Geometry: final body of the model. Coordinates: model frame, mm. Face numbers are marked on the shaded views. A direction names the side the tool comes from. Give positions to 0.01 mm unless a question says otherwise; leave off trailing zeros. Order: outer loops, then holes, each group sorted by start corner. A loop starts at its lowest first (then second) coordinate and runs counter-clockwise, first axis right, second up. Notation, with made-up numbers: M -37,7.5 L -29,7.5 A25 cw -29,23.5 Z; hole C -31,69.5 d1. An arc over 180 degrees is marked long. Use CSV: the item, a comma, the result in double quotes.
```python
from build123d import *

# Parameters (mm, degrees)
PAD_DEPTH       = 4.5
SKETCH001_R     = 3.6
POCKET_DEPTH    = 4.501
POCKET001_DEPTH = 1.5
SKETCH003_R     = 0.6
POCKET002_DEPTH = 3.001
CHAMFER_SIZE    = 0.6


with BuildPart() as part:
    # Sketch → Pad (new body)
    with BuildSketch(Plane.XY):
        with BuildLine():
            ThreePointArc((0, -4.5), (4.5, 0), (0, 4.5))
            Line((0, 4.5), (-26, 4.5))
            ThreePointArc((-26, 4.5), (-29.181981, 3.181981), (-30.5, 0))
            ThreePointArc((-30.5, 0), (-23.829371, -8.693332), (-13.705771, -4.5))
            Line((0, -4.5), (-13.705771, -4.5))
        make_face()
    extrude(amount=PAD_DEPTH)

    # Sketch001 (on Face7 of Pad) → Pocket (cut, through all)
    with BuildSketch(Plane.XY.offset(4.5)):
        Circle(SKETCH001_R)
    extrude(amount=-POCKET_DEPTH, mode=Mode.SUBTRACT)

    # Sketch002 (on Face5 of Pocket) → Pocket001 (cut)
    with BuildSketch(Plane.XY.offset(4.5)):
        with BuildLine():
            ThreePointArc((-14.63696, 1.995305), (-16.5, 0), (-14.63696, -1.995305))
            Line((-14.63696, -1.995305), (0, -3))
            Line((0, 3), (0, -3))
            Line((-14.63696, 1.995305), (0, 3))
        make_face()
    extrude(amount=-POCKET001_DEPTH, mode=Mode.SUBTRACT)

    # Sketch003 (on Face12 of Pocket001) → Pocket002 (cut, through all)
    with BuildSketch(Plane.XY.offset(3)):
        with Locations((-14.5, 0)):
            Circle(SKETCH003_R)
        with Locations((-12.5, 0)):
            Circle(SKETCH003_R)
        with Locations((-10.5, 0)):
            Circle(SKETCH003_R)
        with Locations((-8.5, 0)):
            Circle(SKETCH003_R)
        with Locations((-6.5, 0)):
            Circle(SKETCH003_R)
        with Locations((-4.5, 0)):
            Circle(SKETCH003_R)
    extrude(amount=-POCKET002_DEPTH, mode=Mode.SUBTRACT)

    # Chamfer
    chamfer_edges = [part.edges().sort_by_distance(p)[0] for p in [
        (-23.829371, -8.693332, 4.5),
        (-23.829371, -8.693332, 0),
    ]]
    chamfer(chamfer_edges, length=CHAMFER_SIZE)


solid = part.part
```
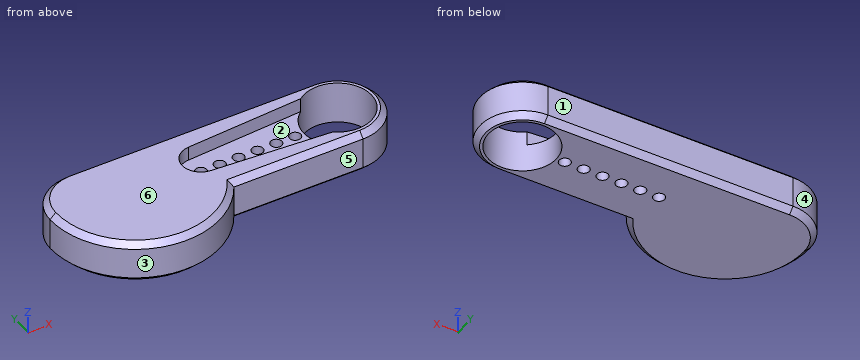
1. Pull-direction query (X, two-part tool) for the marked faces 1, 2, 3 and 4; classes: +X half, -X half, draft (parallel to the pull), parting line (faces both ways), or undercut.
Answer:
face 1,"draft"
face 2,"undercut"
face 3,"parting line"
face 4,"-X half"
2. Section D-D, the plane x = -6.5. Return the cut outline in (y, z), plus the area to 3 significant figures.
Answer:
outline,"M -4.5,0.6 L -3.9,0 L -0.6,0 L -0.6,3 L -2.55,3 L -2.55,4.5 L -3.9,4.5 L -4.5,3.9 Z; M 0.6,0 L 3.9,0 L 4.5,0.6 L 4.5,3.9 L 3.9,4.5 L 2.55,4.5 L 2.55,3 L 0.6,3 Z"
area,"28.5 mm2"
3. Section C-C, the plane x = -1. Return the cut outline in (y, z), plus the area to 3 significant figures.
Answer:
outline,"M -4.5,0.6 L -3.9,0 L -3.46,0 L -3.46,4.5 L -3.9,4.5 L -4.5,3.9 Z; M 3.46,0 L 3.9,0 L 4.5,0.6 L 4.5,3.9 L 3.9,4.5 L 3.46,4.5 Z"
area,"8.66 mm2"
4. Section B-B, the plane x = -10.5. Return the cut outline in (y, z), plus the area to 3 significant figures.
Answer:
outline,"M -4.5,0.6 L -3.9,0 L -0.6,0 L -0.6,3 L -2.28,3 L -2.28,4.5 L -3.9,4.5 L -4.5,3.9 Z; M 0.6,0 L 3.9,0 L 4.5,0.6 L 4.5,3.9 L 3.9,4.5 L 2.28,4.5 L 2.28,3 L 0.6,3 Z"
area,"29.3 mm2"
5. Pin query (flat end, axial travel): pin 1 Ø0.7 at (x, y) = (-4.5, 0) entering from +Z; pin 2 Ø1.4 at (x, y) = (-14.5, 0) entering from +Z; pin 3 Ø2 at (x, z) = (-6.5, 1) entering from -Y. Return the tip coordinate at first contact, or that it passes through.
Answer:
pin 1,"through"
pin 2,"z = 3"
pin 3,"y = -4.5"
6. Reachability of the marked faces 5 and 6 from +Z, -Z, +X, -X, +Y, -Y: full face, straight path, thin tool, end or side. Return the list, or none.
Answer:
face 5,"+Z, -Z, +X, -Y"
face 6,"+Z, +X, -X, +Y, -Y"
7. Section A-A, the plane z = 1.2. Return the cut outline in (x, y), plus the area to 3 significant figures.
Answer:
outline,"M -30.5,0 A9 ccw -13.71,-4.5 L 0,-4.5 A4.5 ccw 0,4.5 L -26,4.5 A4.5 ccw Z; hole C -14.5,0 d1.2; hole C -12.5,0 d1.2; hole C -10.5,0 d1.2; hole C -8.5,0 d1.2; hole C -6.5,0 d1.2; hole C -4.5,0 d1.2; hole C 0,0 d7.2"
area,"302 mm2"
8. Line query: line 1 (Y direction, x = -10.5, z = 1); line 2 (X direction, y = -1.5, z = 2.15); line 3 (X direction, y = 1.25, z = 3.35). Output: solid intervals per line, ascending.
Answer:
line 1,"-4.5 to -0.6, 0.6 to 4.5"
line 2,"-30.37 to -3.27, 3.27 to 4.24"
line 3,"-30.32 to -16.06, 3.38 to 4.32"
